Part model, mm, in its own coordinate system. Face numbers are marked on the shaded views. A direction names the side the tool comes from. Give positions to 0.01 mm unless a question says otherwise; leave off trailing zeros. Write each loop counter-clockwise with the first axis right and the second up, starting at its lowest first coordinate (ties: lowest second). Pieces come first, ordered by that corner, then holes. Notation, with made-up numbers: M 50.5,69.5 L 70.5,69.5 A29 ccw 70.5,94.5 Z; hole C -27.75,59.25 d8. An arc over 180 degrees is marked long. Use a Markdown table: item, result.
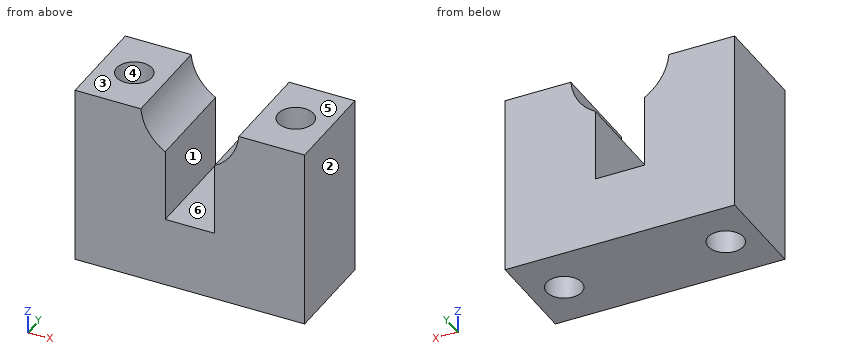
Solid Edge part; units mm, degrees
sketch "Sketch1" plane through (0, 0, 0) normal (0, 0, 1) x (1, 0, 0)
  line L0 (-14, -6) -> (14, -6)
  line L1 (14, -6) -> (14, 6)
  line L2 (14, 6) -> (-14, 6)
  line L3 (-14, 6) -> (-14, -6)
  dimension "D1" = 14
  dimension "D2" = 14
extrude "Ajout_matière_1" add sketch "Sketch1" along normal blind 22
sketch "Sketch2" plane through (0, -6, 10) normal (0, -1, 0) x (1, 0, 0)
  circle A0 centre (0, 12.5) radius 6
extrude "Cutout1" cut sketch "Sketch2" against normal through all
sketch "Sketch3" plane through (0, -6, 10) normal (0, -1, 0) x (1, 0, 0)
  line L0 (-3, -1.5) -> (3, -1.5)
  line L1 (3, -1.5) -> (3, 12.5)
  line L2 (3, 12.5) -> (-3, 12.5)
  line L3 (-3, 12.5) -> (-3, -1.5)
  dimension "D1" = 3
  dimension "D2" = 3
  dimension "D3" = 3
extrude "Cutout2" cut sketch "Sketch3" against normal through all
hole "Perçage_1" at (9.85, 0, 0) direction (0, 0, 1) diameter 4.3 end through all
hole "Hole1" at (-9.85, 0, 0) direction (0, 0, 1) diameter 4.3 end through all
properties material "Plastique ABS, performance moyenne"
1. Cut at A-A, the plane y = 0. Give the cut face in (x, z).
Findings below:
| item | result |
|---|---|
| outline | M -14,0 L -12,0 L -12,22 L -14,22 Z; M -7.7,0 L 7.7,0 L 7.7,22 L 5.98,22 A6 cw 3,17.3 L 3,8.5 L -3,8.5 L -3,17.3 A6 cw -5.98,22 L -7.7,22 Z; M 12,0 L 14,0 L 14,22 L 12,22 Z |
2. Cut at B-B, the plane x = 9.85. Give the cut face in (y, z).
Findings below:
| item | result |
|---|---|
| outline | M -6,0 L -2.15,0 L -2.15,22 L -6,22 Z; M 2.15,0 L 6,0 L 6,22 L 2.15,22 Z |
3. Two-plate mould, pull along X, no slides. Class the marked faces 1, 2, 3 and 4: released by +X, released by -X, zero draft, split by the parting line, or undercut.
Findings below:
| item | result |
|---|---|
| face 1 | undercut |
| face 2 | released by +X |
| face 3 | zero draft |
| face 4 | undercut |
4. Drop flat-ended pins along their axis: P1, Ø2, axis at x = 2.5, z = 15, coming from the +Y side; P2, Ø2.5, axis at x = -9.85, y = 0, coming from the -Z side; P3, Ø5, axis at x = -1, y = 0, coming from the +Z side. Give the stop position or say it passes through.
Findings below:
| item | result |
|---|---|
| P1 | y = 6 |
| P2 | through |
| P3 | z = 17.63 |
5. Cut at C-C, the plane y = 3.5. Give the cut face in (x, z), then the cut area to 3 significant figures.
Findings below:
| item | result |
|---|---|
| outline | M -14,0 L 14,0 L 14,22 L 5.98,22 A6 cw 3,17.3 L 3,8.5 L -3,8.5 L -3,17.3 A6 cw -5.98,22 L -14,22 Z |
| area | 516 mm2 |
6. Drill centre lines: L1, parallel to X at y = 0, z = 8.25; L2, parallel to Y at x = -9.85, z = 5.5; L3, parallel to X at y = -2.25, z = 10.25. Where is each one in solid material? Low to high.
Findings below:
| item | result |
|---|---|
| L1 | -14 to -12, -7.7 to 7.7, 12 to 14 |
| L2 | -6 to -2.15, 2.15 to 6 |
| L3 | -14 to -3, 3 to 14 |
7. Tool access for the marked faces 5 and 6: list every direction of +Z, -Z, +X, -X, +Y, -Y with a clear straight run to the whole face (end or side of a thin tool).
Findings below:
| item | result |
|---|---|
| face 5 | +Z, +X, -X, +Y, -Y |
| face 6 | +Z, +Y, -Y |
8. Cut at D-D, the plane z = 1.5. Give the cut face in (x, y).
Findings below:
| item | result |
|---|---|
| outline | M -14,-6 L 14,-6 L 14,6 L -14,6 Z; hole C -9.85,0 d4.3; hole C 9.85,0 d4.3 |
